The listing builds one solid part. Answer for the finished solid, in the listing's coordinates (mm). Face numbers are marked on the shaded views. A direction names the side the tool comes from. Coordinates: 2 decimals unless noted, no trailing zeros. Loops run counter-clockwise (first coordinate to the right, second up) from the corner with the lowest first, then second, coordinate; pieces in that order, holes last. Notation, with made-up numbers: (48, 1.25) - (97, 1.25) arc R9 ccw to (97, 16.25) - close; hole circle Ø11 at (-0.5, 73). An arc over 180 degrees is marked (long way). Use one line per item in the form item = value. Start each with the question number.
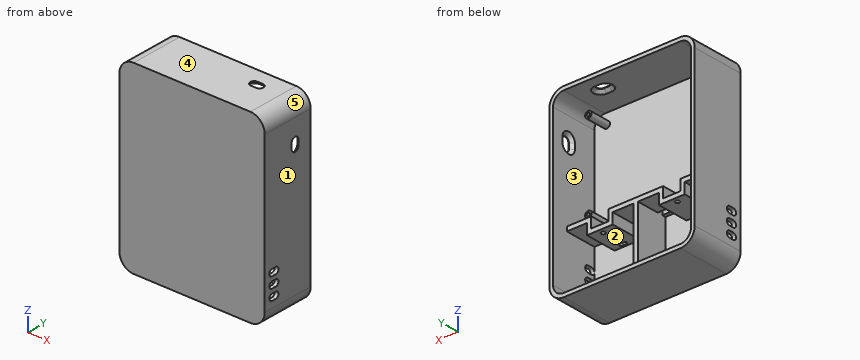
```python
from build123d import *

# Parameters (mm, degrees)
BOSS_EXTRUDE1_DEPTH = 5
BOSS_EXTRUDE2_DEPTH = 30
SKETCH3_R           = 2
CUT_EXTRUDE1_DEPTH  = 126.103956772
BOSS_EXTRUDE3_DEPTH = 50
SKETCH7_R           = 3.0875
SKETCH7_R_2         = 1.5875
BOSS_EXTRUDE4_DEPTH = 20
SKETCH9_W           = 4
SKETCH9_H           = 67.5
BOSS_EXTRUDE5_DEPTH = 30
CUT_EXTRUDE2_DEPTH  = 20
CUT_EXTRUDE3_DEPTH  = 10
CHAMFER1_SIZE       = 3
CUT_EXTRUDE4_DEPTH  = 121.781828103
CHAMFER2_SIZE       = 3


with BuildPart() as part:
    # Sketch1 → Boss-Extrude1 (new body)
    with BuildSketch(Plane(origin=(0, 0, 0), x_dir=(1, 0, 0), z_dir=(0, 1, 0))):
        with BuildLine():
            Line((-55, -82.5), (55, -82.5))
            ThreePointArc((55, -82.5), (62.071067812, -79.571067812), (65, -72.5))
            Line((65, -72.5), (65, 72.5))
            ThreePointArc((65, 72.5), (62.071067812, 79.571067812), (55, 82.5))
            Line((55, 82.5), (-55, 82.5))
            ThreePointArc((-55, 82.5), (-62.071067812, 79.571067812), (-65, 72.5))
            Line((-65, 72.5), (-65, -72.5))
            ThreePointArc((-65, -72.5), (-62.071067812, -79.571067812), (-55, -82.5))
        make_face()
    extrude(amount=BOSS_EXTRUDE1_DEPTH)

    # Sketch2 → Boss-Extrude2 (add)
    with BuildSketch(Plane(origin=(0, 5, 0), x_dir=(1, 0, 0), z_dir=(0, 1, 0))):
        Polygon((-65, 18.5), (-42, 18.5), (-42, 28.5), (-25.74846966, 28.5), (-25.74846966, 18.5), (25.74846966, 18.5), (25.74846966, 28.5), (42, 28.5), (42, 18.5), (65, 18.5), (65, 22.5), (46, 22.5), (46, 32.5), (21.74846966, 32.5), (21.74846966, 22.5), (-21.74846966, 22.5), (-21.74846966, 32.5), (-46, 32.5), (-46, 22.5), (-65, 22.5), align=None)
    extrude(amount=BOSS_EXTRUDE2_DEPTH)

    # Sketch3 → Cut-Extrude1 (cut, through all)
    with BuildSketch(Plane.XY.offset(-18.5)):
        with Locations((35, 30)):
            Circle(SKETCH3_R)
        with Locations((-35, 30)):
            Circle(SKETCH3_R)
        with BuildLine():
            Line((-12.5, 13.50518346), (12.5, 13.50518346))
            ThreePointArc((12.5, 13.50518346), (15.00518346, 11), (12.5, 8.49481654))
            Line((12.5, 8.49481654), (-12.5, 8.49481654))
            ThreePointArc((-12.5, 8.49481654), (-15.00518346, 11), (-12.5, 13.50518346))
        make_face()
        with BuildLine():
            Line((33, 9.98963308), (37, 9.98963308))
            ThreePointArc((37, 9.98963308), (38.49481654, 8.49481654), (37, 7))
            Line((37, 7), (33, 7))
            ThreePointArc((33, 7), (31.50518346, 8.49481654), (33, 9.98963308))
        make_face()
        with BuildLine():
            Line((-33, 9.98963308), (-37, 9.98963308))
            ThreePointArc((-37, 9.98963308), (-38.49481654, 8.49481654), (-37, 7))
            Line((-37, 7), (-33, 7))
            ThreePointArc((-33, 7), (-31.50518346, 8.49481654), (-33, 9.98963308))
        make_face()
    extrude(amount=-CUT_EXTRUDE1_DEPTH, mode=Mode.SUBTRACT)

    # Sketch1_3 → Boss-Extrude3 (add)
    with BuildSketch(Plane(origin=(0, 0, 0), x_dir=(1, 0, 0), z_dir=(0, 1, 0))):
        with BuildLine():
            Line((-68.5, -72.5), (-68.5, 72.5))
            ThreePointArc((-68.5, 72.5), (-64.545941546, 82.045941546), (-55, 86))
            Line((-55, 86), (55, 86))
            ThreePointArc((55, 86), (64.545941546, 82.045941546), (68.5, 72.5))
            Line((68.5, 72.5), (68.5, -72.5))
            ThreePointArc((68.5, -72.5), (64.545941546, -82.045941546), (55, -86))
            Line((55, -86), (-55, -86))
            ThreePointArc((-55, -86), (-64.545941546, -82.045941546), (-68.5, -72.5))
        make_face()
        with BuildLine():
            Line((-55, -82.5), (55, -82.5))
            ThreePointArc((55, -82.5), (62.071067812, -79.571067812), (65, -72.5))
            Line((65, -72.5), (65, 72.5))
            ThreePointArc((65, 72.5), (62.071067812, 79.571067812), (55, 82.5))
            Line((55, 82.5), (-55, 82.5))
            ThreePointArc((-55, 82.5), (-62.071067812, 79.571067812), (-65, 72.5))
            Line((-65, 72.5), (-65, -72.5))
            ThreePointArc((-65, -72.5), (-62.071067812, -79.571067812), (-55, -82.5))
        make_face(mode=Mode.SUBTRACT)
    extrude(amount=BOSS_EXTRUDE3_DEPTH)

    # Sketch7 → Boss-Extrude4 (add)
    # profile 1 of 4: a face of its own
    with BuildSketch(Plane(origin=(0, 5, 0), x_dir=(1, 0, 0), z_dir=(0, 1, 0))):
        with Locations(Location((-53.3075, -72.59, 0), (0, 0, 90))):
            Circle(SKETCH7_R)
        with Locations(Location((-53.3075, -72.59, 0), (0, 0, 270))):
            Circle(SKETCH7_R_2, mode=Mode.SUBTRACT)
    # profile 2 of 4: a face of its own
    with BuildSketch(Plane(origin=(0, 5, 0), x_dir=(1, 0, 0), z_dir=(0, 1, 0))):
        with Locations(Location((53.3725, -72.59, 0), (0, 0, 90))):
            Circle(SKETCH7_R)
        with Locations(Location((53.3725, -72.59, 0), (0, 0, 270))):
            Circle(SKETCH7_R_2, mode=Mode.SUBTRACT)
    # profile 3 of 4: a face of its own
    with BuildSketch(Plane(origin=(0, 5, 0), x_dir=(1, 0, 0), z_dir=(0, 1, 0))):
        with Locations(Location((-53.3075, 8.69, 0), (0, 0, 90))):
            Circle(SKETCH7_R)
        with Locations(Location((-53.3075, 8.69, 0), (0, 0, 270))):
            Circle(SKETCH7_R_2, mode=Mode.SUBTRACT)
    # profile 4 of 4: a face of its own
    with BuildSketch(Plane(origin=(0, 5, 0), x_dir=(1, 0, 0), z_dir=(0, 1, 0))):
        with Locations(Location((53.3725, 8.69, 0), (0, 0, 90))):
            Circle(SKETCH7_R)
        with Locations(Location((53.3725, 8.69, 0), (0, 0, 270))):
            Circle(SKETCH7_R_2, mode=Mode.SUBTRACT)
    extrude(amount=BOSS_EXTRUDE4_DEPTH)

    # Sketch9 → Boss-Extrude5 (add)
    with BuildSketch(Plane(origin=(0, 35, 0), x_dir=(1, 0, 0), z_dir=(0, 1, 0))):
        with Locations((0, 52.25)):
            Rectangle(SKETCH9_W, SKETCH9_H)
    extrude(amount=-BOSS_EXTRUDE5_DEPTH)

    # Sketch11 → Cut-Extrude2 (cut)
    with BuildSketch(Plane.ZY.offset(68.5)):
        with BuildLine():
            Line((-66.522203209, 8), (-66.522203209, 12))
            ThreePointArc((-66.522203209, 12), (-63.522203209, 15), (-60.522203209, 12))
            Line((-60.522203209, 12), (-60.522203209, 8))
            ThreePointArc((-60.522203209, 8), (-63.522203209, 5), (-66.522203209, 8))
        make_face()
        with BuildLine():
            Line((-50.522203209, 8), (-50.522203209, 12))
            ThreePointArc((-50.522203209, 12), (-53.522203209, 15), (-56.522203209, 12))
            Line((-56.522203209, 12), (-56.522203209, 8))
            ThreePointArc((-56.522203209, 8), (-53.522203209, 5), (-50.522203209, 8))
        make_face()
        with BuildLine():
            Line((-40.522203209, 8), (-40.522203209, 12))
            ThreePointArc((-40.522203209, 12), (-43.522203209, 15), (-46.522203209, 12))
            Line((-46.522203209, 12), (-46.522203209, 8))
            ThreePointArc((-46.522203209, 8), (-43.522203209, 5), (-40.522203209, 8))
        make_face()
    cut_extrude2 = extrude(amount=-CUT_EXTRUDE2_DEPTH, mode=Mode.SUBTRACT)

    # Mirror1: Cut-Extrude2 across plane
    add(cut_extrude2.mirror(Plane(origin=(2, 5, -86), x_dir=(0, 0, 1), z_dir=(1, 0, 0))), mode=Mode.SUBTRACT)

    # Sketch12 → Cut-Extrude3 (cut)
    with BuildSketch(Plane(origin=(68.5, 0, 0), x_dir=(0, 0, -1), z_dir=(1, 0, 0))):
        with BuildLine():
            Line((-53, 36.75), (-48, 36.75))
            ThreePointArc((-48, 36.75), (-44.25, 33), (-48, 29.25))
            Line((-48, 29.25), (-53, 29.25))
            ThreePointArc((-53, 29.25), (-56.75, 33), (-53, 36.75))
        make_face()
    extrude(amount=-CUT_EXTRUDE3_DEPTH, mode=Mode.SUBTRACT)

    # Chamfer1
    chamfer1_edges = [part.edges().sort_by_distance(p)[0] for p in [
        (65, 33, 56.75),
        (65, 36.75, 50.5),
        (65, 33, 44.25),
        (65, 29.25, 50.5),
    ]]
    chamfer(chamfer1_edges, length=CHAMFER1_SIZE)

    # Sketch13 → Cut-Extrude4 (cut, through all)
    with BuildSketch(Plane.XY):
        with BuildLine():
            Line((30, 36.75), (35, 36.75))
            ThreePointArc((35, 36.75), (38.75, 33), (35, 29.25))
            Line((35, 29.25), (30, 29.25))
            ThreePointArc((30, 29.25), (26.25, 33), (30, 36.75))
        make_face()
    extrude(amount=CUT_EXTRUDE4_DEPTH, mode=Mode.SUBTRACT)

    # Chamfer2
    chamfer2_edges = [part.edges().sort_by_distance(p)[0] for p in [
        (26.25, 33, 82.5),
        (32.5, 29.25, 82.5),
        (38.75, 33, 82.5),
        (32.5, 36.75, 82.5),
    ]]
    chamfer(chamfer2_edges, length=CHAMFER2_SIZE)


solid = part.part
```
(1) Find the intervals of material crossed by probe 1 along X at (y, z) = (18.5, -56); probe 2 along Z at (x, y) = (17.5, 7); probe 3 along X at (y, z) = (21.5, -21.5), in increasing order. Write a range as from..to.
(2) A cutting plane is placed at D-D (y = 21.5). State how many separate pieces and enclosed holes the cut face has, then the cut area to 3 significant figures.
(3) A cutting plane is placed at B-B (y = 45). Determine the outline of the cut face in (x, z), then the cut area to 3 significant figures.
(4) For the marked faces 1 and 2, determine the directions among +Z, -Z, +X, -X, +Y, -Y from which every point of the face is accessible in a straight line to the end or side of a thin tool.
(5) A cutting plane is placed at C-C (z = 33.5). Determine the outline of the cut face in (x, y).
(6) Determine the mould class of the marked faces 3, 4 and 5 for opening direction X: +X half, -X half, draft (parallel to the pull), parting line (faces both ways), or undercut.
(7) Each of these flat-tipped pins is pushed along its axis until it touches: pin 1 Ø8 at (x, z) = (12, -54) entering from +Y; pin 2 Ø4 at (x, z) = (-53.31, 72.59) entering from +Y; pin 3 Ø5 at (x, z) = (-51.5, -18.5) entering from +Y; pin 4 Ø1 at (x, z) = (-26, -28.5) entering from -Y. Where does it stop, or does it pass through?
(8) A cutting plane is placed at A-A (x = -35). Determine the outline of the cut face in (y, z), then the cut area to 3 significant figures.
Evaluation:
q1.probe_1 = -68.5..-65, -2..2, 65..68.5
q1.probe_2 = -86..-82.5, -22.5..-18.5, 82.5..86
q1.probe_3 = -68.5..-42, -25.75..25.75, 42..68.5
q2.separate_pieces = 5
q2.enclosed_holes = 7
q2.area = 3,050 mm^2
q3.outline = (-68.5, -72.5) arc R13.5 ccw to (-55, -86) - (55, -86) arc R13.5 ccw to (68.5, -72.5) - (68.5, 72.5) arc R13.5 ccw to (55, 86) - (-55, 86) arc R13.5 ccw to (-68.5, 72.5) - close; hole (-65, -72.5) arc R10 ccw to (-55, -82.5) - (55, -82.5) arc R10 ccw to (65, -72.5) - (65, 72.5) arc R10 ccw to (55, 82.5) - (-55, 82.5) arc R10 ccw to (-65, 72.5) - close
q3.area = 2,040 mm^2
q4.face_1 = +Z, -Z, +X, +Y, -Y
q4.face_2 = +Y
q5.outline = (-68.5, 0) - (68.5, 0) - (68.5, 50) - (65, 50) - (65, 5) - (-65, 5) - (-65, 50) - (-68.5, 50) - close
q6.face_3 = undercut
q6.face_4 = draft
q6.face_5 = +X half
q7.pin_1 = 5
q7.pin_2 = 25
q7.pin_3 = 35
q7.pin_4 = 0
q8.outline = (0, -86) - (50, -86) - (50, -82.5) - (5, -82.5) - (5, -32.5) - (7, -32.5) - (7, -28.5) - (5, -28.5) - (5, 82.5) - (50, 82.5) - (50, 86) - (0, 86) - close; (9.99, -32.5) - (28, -32.5) - (28, -28.5) - (9.99, -28.5) - close; (32, -32.5) - (35, -32.5) - (35, -28.5) - (32, -28.5) - close
q8.area = 1,270 mm^2
